Source: CAD feature listing. Evaluate the final solid. Frame: model axes, mm. A direction names the side the tool comes from. Give positions to 0.01 mm unless a question says otherwise; leave off trailing zeros. Order: outer loops, then holes, each group sorted by start corner. A loop starts at its lowest first (then second) coordinate and runs counter-clockwise, first axis right, second up. Notation, with made-up numbers: M 84.5,36 L 143.5,36 A25 ccw 143.5,73 Z; hole C 76.5,34.25 d3. An arc over 180 degrees is marked long. Return JSON: item names as keys, results as strings.
Autodesk Fusion 360 part; units mm, degrees
sketch "Sketch1" plane through (0, 0, 0) normal (0, 0, 1) x (1, 0, 0) in component "Top Cover Plate"
  line L0 (0, 0) -> (183.6, 0)
  line L1 (183.6, 0) -> (183.6, 203.6)
  line L2 (183.6, 203.6) -> (0, 203.6)
  line L3 (0, 203.6) -> (0, 0)
  dimension "d1" = 183.6
  dimension "d2" = 203.6
extrude "Extrude1" add sketch "Sketch1" along normal blind 5 in component "Top Cover Plate"
fillet "Fillet1" radius 12 4 edges at (183.6, 0, 2.5) (0, 0, 2.5) (183.6, 203.6, 2.5) (0, 203.6, 2.5) in component "Top Cover Plate"
sketch "Sketch2" plane through (0, 0, 5) normal (0, 0, 1) x (-1, 0, 0) in component "Top Cover Plate"
  arc A0 (-12, -203.6) -> (0, -191.6) centre (-12, -191.6) ccw
  line L0 (0, -191.6) -> (0, -12)
  arc A1 (0, -12) -> (-12, 0) centre (-12, -12) ccw
  line L1 (-12, 0) -> (-171.6, 0)
  arc A2 (-171.6, 0) -> (-183.6, -12) centre (-171.6, -12) ccw
  line L2 (-183.6, -12) -> (-183.6, -191.6)
  arc A3 (-183.6, -191.6) -> (-171.6, -203.6) centre (-171.6, -191.6) ccw
  line L3 (-171.6, -203.6) -> (-12, -203.6)
  line L4 (0, -195.8) -> (-183.6, -195.8) construction
  line L5 (0, -7.8) -> (-183.6, -7.8) construction
  line L6 (-7.8, -203.6) -> (-7.8, 0) construction
  line L7 (-175.8, -203.6) -> (-175.8, 0) construction
  circle A4 centre (-7.8, -195.8) radius 1.75
  circle A5 centre (-175.8, -195.8) radius 1.75
  circle A6 centre (-7.8, -7.8) radius 1.75
  circle A7 centre (-175.8, -7.8) radius 1.75
  dimension "d7" = 7.8
  dimension "d8" = 7.8
  dimension "d9" = 7.8
  dimension "d10" = 7.8
  dimension "d11" = 3.5
  dimension "d12" = 3.5
  dimension "d13" = 3.5
  dimension "d14" = 3.5
extrude "Extrude2" cut sketch "Sketch2" against normal up to surface (5 mm away) contours A4 | A5 | A6 | A7 in component "Top Cover Plate"
sketch "Sketch3" plane through (0, 0, 5) normal (0, 0, 1) x (-1, 0, 0) in component "Top Cover Plate"
  circle A0 centre (-175.8, -195.8) radius 1.75
  circle A1 centre (-7.8, -7.8) radius 1.75
  circle A2 centre (-7.8, -195.8) radius 1.75
  circle A3 centre (-175.8, -7.8) radius 1.75
  arc A4 (-12, -203.6) -> (0, -191.6) centre (-12, -191.6) ccw
  line L0 (0, -191.6) -> (0, -12)
  arc A5 (0, -12) -> (-12, 0) centre (-12, -12) ccw
  line L1 (-12, 0) -> (-171.6, 0)
  arc A6 (-171.6, 0) -> (-183.6, -12) centre (-171.6, -12) ccw
  line L2 (-183.6, -12) -> (-183.6, -191.6)
  arc A7 (-183.6, -191.6) -> (-171.6, -203.6) centre (-171.6, -191.6) ccw
  line L3 (-171.6, -203.6) -> (-12, -203.6)
  line L4 (-91.8, -203.6) -> (-91.8, 0) construction
  line L5 (0, -101.8) -> (-183.6, -101.8) construction
  line L6 (-156.8, -176.8) -> (-26.8, -176.8)
  line L7 (-26.8, -176.8) -> (-26.8, -26.8)
  line L8 (-26.8, -26.8) -> (-156.8, -26.8)
  line L9 (-156.8, -26.8) -> (-156.8, -176.8)
  line L10 (-156.8, -176.8) -> (-26.8, -26.8) construction
  line L11 (-26.8, -176.8) -> (-156.8, -26.8) construction
  point P0 (-91.8, -101.8)
  dimension "d17" = 130
  dimension "d18" = 150
extrude "Extrude3" cut sketch "Sketch3" against normal up to surface (5 mm away) contours L6 L7 L8 L9 in component "Top Cover Plate"
fillet "Fillet2" radius 5 4 edges at (26.8, 26.8, 2.5) (26.8, 176.8, 2.5) (156.8, 176.8, 2.5) (156.8, 26.8, 2.5) in component "Top Cover Plate"
component "Top Cover Plate" placed x (1, 0, 0) y (0, 1, 0) z (0, 0, 1) at (0, 0, 0)
1. Draft query along Y for faces 3 (the face through (91, 0, 2)), 4 (the face through (93, 203.6, 2)), 5 (the face through (28.23, 175.3, 2.46)). Return one class per face: pulls with the +Y half, pulls with the -Y half, needs draft (parallel to the pull), parting line crosses it, or undercut.
Evaluation:
{"face 3": "pulls with the -Y half", "face 4": "pulls with the +Y half", "face 5": "undercut"}
2. Section query C-C (z = 3.65). Return loops of the section in (x, y), then the cut area to 3 significant figures.
Evaluation:
{"outline": "M 0,12 A12 ccw 12,0 L 171.6,0 A12 ccw 183.6,12 L 183.6,191.6 A12 ccw 171.6,203.6 L 12,203.6 A12 ccw 0,191.6 Z; hole C 7.8,7.8 d3.5; hole C 7.8,195.8 d3.5; hole M 26.8,31.8 A5 ccw 31.8,26.8 L 151.8,26.8 A5 ccw 156.8,31.8 L 156.8,171.8 A5 ccw 151.8,176.8 L 31.8,176.8 A5 ccw 26.8,171.8 Z; hole C 175.8,7.8 d3.5; hole C 175.8,195.8 d3.5", "area": "17,700 mm^2"}
3. Ray query, probe 1 along X at (y, z) = (124.5, 4.6); probe 2 along Y at (x, z) = (175.8, 1.85); probe 3 along X at (y, z) = (195.8, 3.25). Return the intervals inside material, ascending.
Evaluation:
{"probe 1": "x = 0 to 26.8, 156.8 to 183.6", "probe 2": "y = 0.76 to 6.05, 9.55 to 194.05, 197.55 to 202.84", "probe 3": "x = 0.76 to 6.05, 9.55 to 174.05, 177.55 to 182.84"}
4. Section query B-B (y = 120). Return loops of the section in (x, z), then the cut area to 3 significant figures.
Evaluation:
{"outline": "M 0,0 L 26.8,0 L 26.8,5 L 0,5 Z; M 156.8,0 L 183.6,0 L 183.6,5 L 156.8,5 Z", "area": "268 mm^2"}
5. Section query A-A (x = 65.5). Return loops of the section in (y, z).
Evaluation:
{"outline": "M 0,0 L 26.8,0 L 26.8,5 L 0,5 Z; M 176.8,0 L 203.6,0 L 203.6,5 L 176.8,5 Z"}
6. Set-up query: faces 1 (the face through (183.6, 101, 2)), 2 (the face through (155.37, 28.3, 2.46)). Return all of +Z, -Z, +X, -X, +Y, -Y with unobstructed straight access to the full face (end or side cutting, diameter ignored); none if empty.
Evaluation:
{"face 1": "+Z, -Z, +X, +Y, -Y", "face 2": "+Z, -Z"}
7. First-contact query: pin 1 (5.5 mm diameter, centred on x = 7.8, y = 195.8, fed in from +Z). Flat tip, straight axial feed; report the tip coordinate or a pass-through.
Evaluation:
{"pin 1": "stops at z = 5"}
